```python
from build123d import *

# Parameters (mm, degrees)
F1_DEPTH = 12.192
F3_DEPTH = 20.321
F4_R     = 9.525
F5_DEPTH = 6.096
F7_D     = 4.2164


with BuildPart() as f1:
    # F0 (on Top) → F1 (new body)
    with BuildSketch(Plane.XY):
        with BuildLine():
            ThreePointArc((0, 6.5786), (6.5786, 0), (0, -6.5786))
            Line((0, -6.5786), (0, -15.24))
            Line((0, -15.24), (13.97, -15.24))
            Line((13.97, -15.24), (20.32, -8.89))
            Line((20.32, -8.89), (20.32, 8.89))
            Line((20.32, 8.89), (13.97, 15.24))
            Line((13.97, 15.24), (0, 15.24))
            Line((0, 15.24), (0, 6.5786))
        make_face()
    extrude(amount=F1_DEPTH)

    # F2 (on face) → F3 (cut, through all)
    with BuildSketch(Plane(origin=(0, 0, 0), x_dir=(0, -1, 0), z_dir=(-1, 0, 0))):
        Polygon((-6.096, 6.096), (-15.24, 6.096), (-15.24, -9.260692), (15.24, -9.260692), (15.24, 6.096), (6.096, 6.096), (6.096, -2.733779), (-6.096, -2.733779), align=None)
    extrude(amount=-F3_DEPTH, mode=Mode.SUBTRACT)

    # F4 (on face) → F5 (cut, through all)
    with BuildSketch(Plane.XY.offset(12.192)):
        Circle(F4_R)
    extrude(amount=-F5_DEPTH, mode=Mode.SUBTRACT)

    # F7 (through all)
    with Locations(Plane.XY.offset(12.192)):
        with Locations((11.43, 10.795), (11.43, -10.795)):
            Hole(F7_D / 2)


solid = f1.part
```
Input: part model. Units: mm. Frame: model coordinates. A direction names the side the tool comes from. Give positions to 0.01 mm unless a question says otherwise; leave off trailing zeros. Order: outer loops, then holes, each group sorted by start corner. A loop starts at its lowest first (then second) coordinate and runs counter-clockwise, first axis right, second up.
1. Reachability of faces 1 (the flat face through (11, -6.096, 3)), 2 (the flat face through (8, 0, 6.096)), 3 (the flat face through (8, 11, 6.096)) from +Z, -Z, +X, -X, +Y, -Y: full face, straight path, thin tool, end or side. Return the list, or none.
Derived:
face 1: -Z, +X, -X, -Y
face 2: +Z, -X
face 3: -Z, +X, -X, +Y
2. Pin query (flat end, axial travel): pin 1 (4.5 mm diameter, centred on x = 7, y = -11, fed in from -Z); pin 2 (6.5 mm diameter, centred on x = 8.5, z = 4, fed in from +Y); pin 3 (6 mm diameter, centred on y = -3, z = 7.5, fed in from -X); pin 4 (1.5 mm diameter, centred on x = 7.5, y = -4, fed in from +Z). Return the tip coordinate at first contact, or that it passes through.
Derived:
pin 1: stops at z = 6.1
pin 2: stops at y = 15.24
pin 3: stops at x = 3.37
pin 4: stops at z = 6.1
3. Mould query, pull axis Y, two halves, no side actions, for faces 4 (the flat face through (17.1, -12.11, 9.1)), 5 (the cylindrical face through (11.887, -12.853, 9.101)), 6 (the flat face through (8, -11, 6.096)). Classes: released by +Y, released by -Y, zero draft, split by the parting line, or undercut.
Derived:
face 4: released by -Y
face 5: undercut
face 6: zero draft
4. Section B-B on y = 12.5. Return the cut outline in (x, z), and give its area (3 significant figures).
Derived:
outline: (0, 6.1) - (10.19, 6.1) - (10.19, 12.19) - (0, 12.19) - close; (12.67, 6.1) - (16.71, 6.1) - (16.71, 12.19) - (12.67, 12.19) - close
area: 86.7 mm2
5. Section A-A on x = 11.43. Return the cut outline in (y, z).
Derived:
outline: (-15.24, 6.1) - (-12.9, 6.1) - (-12.9, 12.19) - (-15.24, 12.19) - close; (-8.69, 6.1) - (-6.1, 6.1) - (-6.1, 0) - (6.1, 0) - (6.1, 6.1) - (8.69, 6.1) - (8.69, 12.19) - (-8.69, 12.19) - close; (12.9, 6.1) - (15.24, 6.1) - (15.24, 12.19) - (12.9, 12.19) - close
6. Material intervals for L1, parallel to Y at x = 11.43, z = 10.5; L2, parallel to Y at x = 10.5, z = 1.5; L3, parallel to Z at x = 6.5, y = 4.5, sorted ascending.
Derived:
L1: y = -15.24 to -12.9, -8.69 to 8.69, 12.9 to 15.24
L2: y = -6.1 to 6.1
L3: z = 0 to 6.1
7. Section C-C on x = 18.25. Return the cut outline in (y, z), and give its area (3 significant figures).
Derived:
outline: (-10.96, 6.1) - (-6.1, 6.1) - (-6.1, 0) - (6.1, 0) - (6.1, 6.1) - (10.96, 6.1) - (10.96, 12.19) - (-10.96, 12.19) - close
area: 208 mm2
8. Section D-D on z = 7. Return the cut outline in (x, y) (3 decimals), and give its area (3 significant figures).
Derived:
outline: (0, -15.24) - (13.97, -15.24) - (20.32, -8.89) - (20.32, 8.89) - (13.97, 15.24) - (0, 15.24) - (0, 9.525) arc R9.525 cw to (0, -9.525) - close; hole circle Ø4.216 at (11.43, -10.795); hole circle Ø4.216 at (11.43, 10.795)
area: 409 mm2
